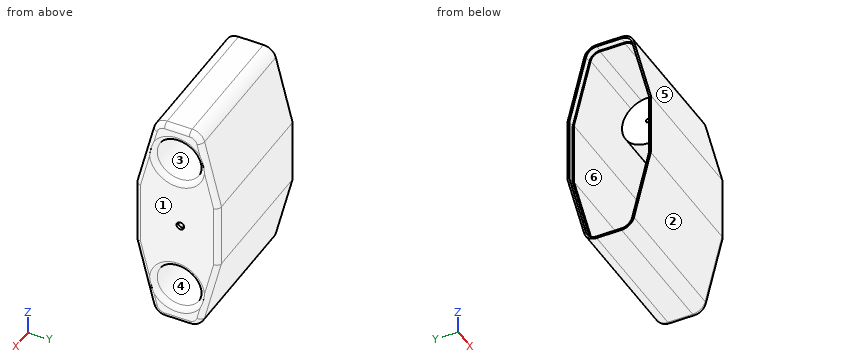
```python
from build123d import *

# Parameters (mm, degrees)
BOSS_EXTRUDE1_DEPTH = 110
SKETCH2_R           = 17.5
CUT_EXTRUDE1_DEPTH  = 50
FILLET1_R           = 10
SHELL1_T            = -2.5
CUT_EXTRUDE4_DEPTH  = 5
FILLET2_R           = 4
SKETCH5_R           = 3
CUT_EXTRUDE5_DEPTH  = 20
SKETCH6_R           = 1.5
CUT_EXTRUDE6_DEPTH  = 20


with BuildPart() as part:
    # Sketch1 → Boss-Extrude1 (new body)
    with BuildSketch(Plane(origin=(0, 0, 0), x_dir=(0, 0, -1), z_dir=(1, 0, 0))):
        Polygon((-25, 25), (-85, 10), (-85, -25), (-25, -40), (25, -40), (85, -25), (85, 10), (25, 25), align=None)
    extrude(amount=-BOSS_EXTRUDE1_DEPTH)

    # Sketch2 → Cut-Extrude1 (cut)
    with BuildSketch(Plane(origin=(0, 0, 0), x_dir=(0, 0, -1), z_dir=(1, 0, 0))):
        with Locations((-55.041193262, -7.5)):
            Circle(SKETCH2_R)
    cut_extrude1 = extrude(amount=-CUT_EXTRUDE1_DEPTH, mode=Mode.SUBTRACT)

    # Fillet1
    fillet1_edges = [part.edges().sort_by_distance(p)[0] for p in [
        (-55, 10, -85),
        (-55, -25, -85),
        (-55, -25, 85),
        (-55, 10, 85),
    ]]
    fillet(fillet1_edges, radius=FILLET1_R)

    # Mirror1: Cut-Extrude1 across plane
    add(cut_extrude1.mirror(Plane.XY), mode=Mode.SUBTRACT)

    # Shell1
    shell1_openings = [part.faces().sort_by_distance(p)[0] for p in [
        (-110, -7.5, 0),
    ]]
    offset(amount=SHELL1_T, openings=shell1_openings, kind=Kind.INTERSECTION)

    # Sketch4 → Cut-Extrude4 (cut)
    with BuildSketch(Plane.ZY.offset(110)):
        with BuildLine():
            Line((-24.692235936, 23.5), (24.692235936, 23.5))
            Line((24.692235936, 23.5), (76.819017188, 10.468304687))
            ThreePointArc((76.819017188, 10.468304687), (81.623972971, 7.468623928), (83.5, 2.123887516))
            Line((83.5, 2.123887516), (83.5, -2.844969352))
            Line((83.5, -2.844969352), (83.5, -17.097430261))
            ThreePointArc((83.5, -17.097430261), (81.771400928, -22.367488253), (77.138058264, -25.416045575))
            Line((77.138058264, -25.416045575), (25.028869166, -38.5))
            Line((25.028869166, -38.5), (-24.692235936, -38.5))
            Line((-24.692235936, -38.5), (-77.034521995, -25.444807466))
            ThreePointArc((-77.034521995, -25.444807466), (-81.692018142, -22.419765778), (-83.5, -17.168637406))
            Line((-83.5, -17.168637406), (-83.5, -2.807764064))
            Line((-83.5, -2.807764064), (-83.5, 2.192235936))
            ThreePointArc((-83.5, 2.192235936), (-81.723124679, 7.497578438), (-76.981950719, 10.468304687))
            Line((-76.981950719, 10.468304687), (-24.692235936, 23.5))
        make_face()
        with BuildLine():
            Line((-24.692235936, 22.5), (24.692235936, 22.5))
            Line((24.692235936, 22.5), (76.819017188, 9.468304687))
            ThreePointArc((76.819017188, 9.468304687), (80.911540785, 6.807827506), (82.5, 2.192235936))
            Line((82.5, 2.192235936), (82.5, -17.192235936))
            ThreePointArc((82.5, -17.192235936), (80.911540785, -21.807827506), (76.819017188, -24.468304687))
            Line((76.819017188, -24.468304687), (24.692235936, -37.5))
            Line((24.692235936, -37.5), (-24.692235936, -37.5))
            Line((-24.692235936, -37.5), (-76.819017188, -24.468304687))
            ThreePointArc((-76.819017188, -24.468304687), (-80.911540785, -21.807827506), (-82.5, -17.192235936))
            Line((-82.5, -17.192235936), (-82.5, 2.192235936))
            ThreePointArc((-82.5, 2.192235936), (-80.911540785, 6.807827506), (-76.819017188, 9.468304687))
            Line((-76.819017188, 9.468304687), (-24.692235936, 22.5))
        make_face(mode=Mode.SUBTRACT)
    extrude(amount=-CUT_EXTRUDE4_DEPTH, mode=Mode.SUBTRACT)

    # Fillet2
    # the kernel refuses this fillet: 4 mm, written as the material it takes off along each edge
    with BuildSketch(Plane(origin=(0, 27.42535625, 15.298574999), x_dir=(-1, 0, 0), z_dir=(0, -0.2425356250363329, 0.970142500145332))) as fillet2_piece_1:
        with BuildLine():
            CenterArc((FILLET2_R, FILLET2_R), FILLET2_R, 180, 90)
            Line((0, FILLET2_R), (0, 0))
            Line((0, 0), (FILLET2_R, 0))
        make_face()
    extrude(amount=64.03882032, mode=Mode.SUBTRACT)
    with BuildSketch(Plane(origin=(0, 25, -35), x_dir=(0, -1, 0), z_dir=(0, 0, 1)), Plane(origin=(0, -40, 35), x_dir=(0, 1, 0), z_dir=(0, 0, -1))) as fillet2_piece_2:
        with BuildLine():
            CenterArc((FILLET2_R, -FILLET2_R), FILLET2_R, 90, 90)
            Line((0, -FILLET2_R), (0, 0))
            Line((0, 0), (FILLET2_R, 0))
        make_face()
    extrude(amount=70, mode=Mode.SUBTRACT)
    with BuildSketch(Plane(origin=(0, -7.5, 55.041193262), x_dir=(0, 0, -1), z_dir=(0, -1, 0))) as fillet2_piece_3:
        with BuildLine():
            CenterArc((17.5 + FILLET2_R, -FILLET2_R), FILLET2_R, 90, 90)
            Line((17.5, -FILLET2_R), (17.5, 0))
            Line((17.5, 0), (17.5 + FILLET2_R, 0))
        make_face()
    revolve(axis=Axis((0, -7.5, 55.041193262), (1, 0, 0)), mode=Mode.SUBTRACT)
    with BuildSketch(Plane(origin=(0, 2.192235936, 85), x_dir=(0, 0, -1), z_dir=(0, -1, 0)), Plane(origin=(0, -17.192235936, -85), x_dir=(0, 0, 1), z_dir=(0, 1, 0))) as fillet2_piece_4:
        with BuildLine():
            CenterArc((FILLET2_R, -FILLET2_R), FILLET2_R, 90, 90)
            Line((0, -FILLET2_R), (0, 0))
            Line((0, 0), (FILLET2_R, 0))
        make_face()
    extrude(amount=19.384471872, mode=Mode.SUBTRACT)
    with BuildSketch(Plane(origin=(0, -26.893660937, 77.42535625), x_dir=(0, 0.970142500145332, -0.24253562503633308), z_dir=(0, -0.24253562503633302, -0.9701425001453319)), Plane(origin=(0, 11.893660937, -77.42535625), x_dir=(0, -0.9701425001453319, 0.24253562503633322), z_dir=(0, 0.24253562503633322, 0.9701425001453319)), Plane(origin=(0, -42.42535625, -15.298574999), x_dir=(0, 0.9701425001453319, 0.2425356250363329), z_dir=(0, 0.24253562503633294, -0.970142500145332))) as fillet2_piece_5:
        with BuildLine():
            CenterArc((FILLET2_R, -FILLET2_R), FILLET2_R, 90, 90)
            Line((0, -FILLET2_R), (0, 0))
            Line((0, 0), (FILLET2_R, 0))
        make_face()
    extrude(amount=64.03882032, mode=Mode.SUBTRACT)
    with BuildSketch(Plane(origin=(0, 2.192235936, 75), x_dir=(0, 0.970142500145332, 0.2425356250363322), z_dir=(0, 0.2425356250363322, -0.970142500145332))) as fillet2_piece_6:
        with BuildLine():
            CenterArc((10 - FILLET2_R, -FILLET2_R), FILLET2_R, 0, 90)
            Line((10, -FILLET2_R), (10, 0))
            Line((10, 0), (10 - FILLET2_R, 0))
        make_face()
    revolve(axis=Axis((0, 2.192235936, 75), (1, 0, 0)), revolution_arc=75.963756532, mode=Mode.SUBTRACT)
    with BuildSketch(Plane(origin=(0, -17.192235936, 75), x_dir=(0, 0, 1), z_dir=(0, 1, 0))) as fillet2_piece_7:
        with BuildLine():
            CenterArc((10 - FILLET2_R, -FILLET2_R), FILLET2_R, 0, 90)
            Line((10, -FILLET2_R), (10, 0))
            Line((10, 0), (10 - FILLET2_R, 0))
        make_face()
    revolve(axis=Axis((0, -17.192235936, 75), (1, 0, 0)), revolution_arc=75.963756532, mode=Mode.SUBTRACT)
    with BuildSketch(Plane(origin=(0, 2.192235936, -75), x_dir=(0, 0.9701425001453317, -0.2425356250363336), z_dir=(0, 0.2425356250363336, 0.9701425001453317))) as fillet2_piece_8:
        with BuildLine():
            CenterArc((10 - FILLET2_R, FILLET2_R), FILLET2_R, 270, 90)
            Line((10, FILLET2_R), (10, 0))
            Line((10, 0), (10 - FILLET2_R, 0))
        make_face()
    revolve(axis=Axis((0, 2.192235936, -75), (-1, 0, 0)), revolution_arc=75.963756532, mode=Mode.SUBTRACT)
    with BuildSketch(Plane(origin=(0, -17.192235936, -75), x_dir=(0, 0, -1), z_dir=(0, 1, 0))) as fillet2_piece_9:
        with BuildLine():
            CenterArc((10 - FILLET2_R, FILLET2_R), FILLET2_R, 270, 90)
            Line((10, FILLET2_R), (10, 0))
            Line((10, 0), (10 - FILLET2_R, 0))
        make_face()
    revolve(axis=Axis((0, -17.192235936, -75), (-1, 0, 0)), revolution_arc=75.963756532, mode=Mode.SUBTRACT)
    with BuildSketch(Plane(origin=(0, -7.5, -55.041193262), x_dir=(0, 0, 1), z_dir=(0, -1, 0))) as fillet2_piece_10:
        with BuildLine():
            CenterArc((17.5 + FILLET2_R, FILLET2_R), FILLET2_R, 180, 90)
            Line((17.5, FILLET2_R), (17.5, 0))
            Line((17.5, 0), (17.5 + FILLET2_R, 0))
        make_face()
    revolve(axis=Axis((0, -7.5, -55.041193262), (-1, 0, 0)), mode=Mode.SUBTRACT)

    # Sketch5 → Cut-Extrude5 (cut)
    with BuildSketch(Plane(origin=(0, 0, 0), x_dir=(0, 0, -1), z_dir=(1, 0, 0))):
        with Locations((0, -5)):
            Circle(SKETCH5_R)
    extrude(amount=-CUT_EXTRUDE5_DEPTH, mode=Mode.SUBTRACT)

    # Sketch6 → Cut-Extrude6 (cut)
    with BuildSketch(Plane(origin=(-50, 0, 0), x_dir=(0, 0, -1), z_dir=(1, 0, 0))):
        with Locations((-55.041193262, -7.5)):
            Circle(SKETCH6_R)
    cut_extrude6 = extrude(amount=-CUT_EXTRUDE6_DEPTH, mode=Mode.SUBTRACT)

    # Mirror3: Cut-Extrude6 across plane
    add(cut_extrude6.mirror(Plane.XY), mode=Mode.SUBTRACT)


solid = part.part
```
Verification items for the finished model (mm, model axes). Face numbers are marked on the shaded views. A direction names the side the tool comes from. Round coordinates to 2 decimals unless told otherwise and drop trailing zeros. Order: outer loops, then holes, each group sorted by start corner. A loop starts at its lowest first (then second) coordinate and runs counter-clockwise, first axis right, second up.
1) Depth check by flat-ended pin: pin 1 (20 mm diameter, centred on y = -7.5, z = -52.5, fed in from -X); pin 2 (2 mm diameter, centred on y = 17.5, z = 8.5, fed in from -X); pin 3 (3 mm diameter, centred on y = 13, z = 64.5, fed in from +X); pin 4 (5 mm diameter, centred on y = -5, z = 0, fed in from +X). Enter the tip coordinate at first touch or a pass-through.
Geometry says:
pin 1: stops at x = -52.5
pin 2: stops at x = -2.5
pin 3: stops at x = -0.02
pin 4: passes through
2) Draft check along Y on the marked faces 1, 2, 3 and 4. Enter one of: +Y half, -Y half, draft (parallel to the pull), parting line (faces both ways), or undercut.
Geometry says:
face 1: draft
face 2: -Y half
face 3: undercut
face 4: undercut
3) Material ranges on line 1 (Z direction, x = -30, y = -7); line 2 (Y direction, x = -24, z = -24.5); line 3 (Z direction, x = -104, y = -1), recorded low to high.
Geometry says:
line 1: z = -85 to -82.5, -75.03 to -72.53, -37.55 to -35.05, 35.05 to 37.55, 72.53 to 75.03, 82.5 to 85
line 2: y = -40 to -37.5, 22.5 to 25
line 3: z = -85 to -82.5, 82.5 to 85
4) Cross-section at B-B, the plane z = 0. Record the cut outline in (x, y), plus the area to 3 significant figures.
Geometry says:
outline: (-110, -40) - (-4, -40) arc R4 ccw to (0, -36) - (0, -8) - (-2.5, -8) - (-2.5, -37.5) - (-105, -37.5) - (-105, -38.5) - (-110, -38.5) - close; (-110, 23.5) - (-105, 23.5) - (-105, 22.5) - (-2.5, 22.5) - (-2.5, -2) - (0, -2) - (0, 21) arc R4 ccw to (-4, 25) - (-110, 25) - close
area: 668 mm2
5) Tool access check on the marked faces 5 and 6. Record the directions out of +Z, -Z, +X, -X, +Y, -Y that give a thin tool (end or side, any length) a straight path to the whole face; none if there is none.
Geometry says:
face 5: +Z, +X, -X, -Y
face 6: -X
6) Cross-section at A-A, the plane x = -12. Record the cut outline in (y, z), plus the area to 3 significant figures.
Geometry says:
outline: (-40, -25) - (-26.89, -77.43) arc R10 ccw to (-17.19, -85) - (2.19, -85) arc R10 ccw to (11.89, -77.43) - (25, -25) - (25, 25) - (11.89, 77.43) arc R10 ccw to (2.19, 85) - (-17.19, 85) arc R10 ccw to (-26.89, 77.43) - (-40, 25) - close; circle Ø40 at (-7.5, -55.04); circle Ø40 at (-7.5, 55.04); hole (-37.5, -24.69) - (-24.47, -76.82) arc R7.5 ccw to (-17.19, -82.5) - (2.19, -82.5) arc R7.5 ccw to (9.47, -76.82) - (22.5, -24.69) - (22.5, 24.69) - (9.47, 76.82) arc R7.5 ccw to (2.19, 82.5) - (-17.19, 82.5) arc R7.5 ccw to (-24.47, 76.82) - (-37.5, 24.69) - close; hole circle Ø35 at (-7.5, -55.04); hole circle Ø35 at (-7.5, 55.04)
area: 1,590 mm2
7) Cross-section at C-C, the plane x = -66. Record the cut outline in (y, z).
Geometry says:
outline: (-40, -25) - (-26.89, -77.43) arc R10 ccw to (-17.19, -85) - (2.19, -85) arc R10 ccw to (11.89, -77.43) - (25, -25) - (25, 25) - (11.89, 77.43) arc R10 ccw to (2.19, 85) - (-17.19, 85) arc R10 ccw to (-26.89, 77.43) - (-40, 25) - close; hole (-37.5, -24.69) - (-24.47, -76.82) arc R7.5 ccw to (-17.19, -82.5) - (2.19, -82.5) arc R7.5 ccw to (9.47, -76.82) - (22.5, -24.69) - (22.5, 24.69) - (9.47, 76.82) arc R7.5 ccw to (2.19, 82.5) - (-17.19, 82.5) arc R7.5 ccw to (-24.47, 76.82) - (-37.5, 24.69) - close
